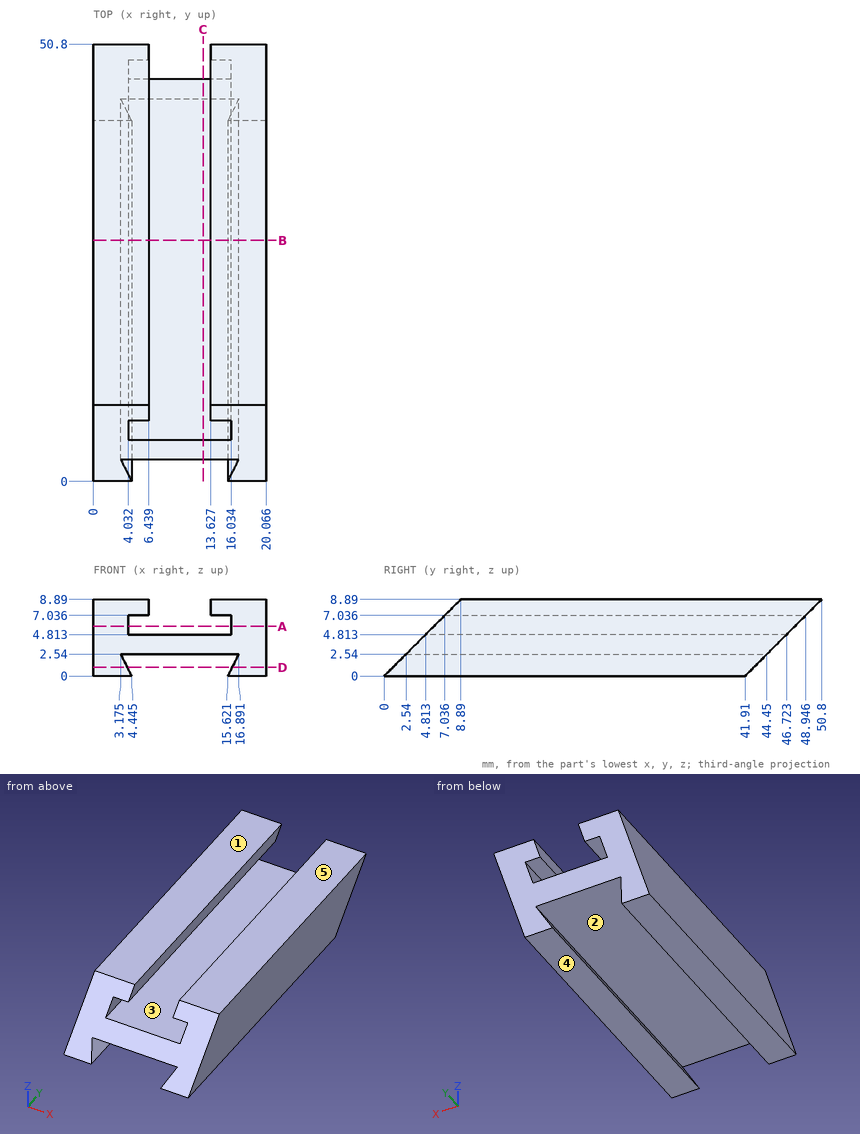
Source: three-view drawing plus pictorial views. Frame: mm from the lowest corner of the part. A direction names the side the tool comes from. Round coordinates to 2 decimals unless told otherwise and drop trailing zeros. Write each loop counter-clockwise with the first axis right and the second up, starting at its lowest first coordinate (ties: lowest second). Pieces come first, ordered by that corner, then holes. Notation, with made-up numbers: M -12.5,40.5 L -8.5,40.5 A26 ccw -8.5,70.5 Z; hole C 30.5,73.5 d3. An arc over 180 degrees is marked long. One line per item, written item: value. Start each with the question number.
Item 1: Section query D-D (z = 1). Return the cut outline in (x, y) (1 decimal), plus the area to 3 significant figures.
Item 2: Section query C-C (x = 12.75). Return the cut outline in (y, z).
Item 3: Section query B-B (y = 28). Return the cut outline in (x, z) (1 decimal).
Item 4: Section query A-A (z = 5.75). Return the cut outline in (x, y), plus the area to 3 significant figures.
Item 5: Pin query (flat end, axial travel): pin 1 (4 mm diameter, centred on x = 9.5, y = 19.5, fed in from +Z); pin 2 (1.5 mm diameter, centred on x = 15.5, z = 7.5, fed in from +Y). Return the tip coordinate at first contact, or that it passes through.
Item 6: Ray query, L1, parallel to Z at x = 15.5, y = 18.5; L2, parallel to X at y = 18, z = 5.25; L3, parallel to Z at x = 4.25, y = 8.5 (1 decimal). Return the intervals inside material, ascending. Write a range as from..to.
Item 7: Mould query, pull axis Z, two halves, no side actions, for the marked faces 3, 4 and 5. Classes: pulls with the +Z half, pulls with the -Z half, needs draft (parallel to the pull), parting line crosses it, or undercut.
Item 8: Set-up query: the marked faces 1 and 2. Return all of +Z, -Z, +X, -X, +Y, -Y with unobstructed straight access to the full face (end or side cutting, diameter ignored); none if empty.
Result set:
1. outline: M 0,1 L 3.9,1 L 3.9,42.9 L 0,42.9 Z; M 16.1,1 L 20.1,1 L 20.1,42.9 L 16.1,42.9 Z
1. area: 331 mm²
2. outline: M 2.54,2.54 L 44.45,2.54 L 46.72,4.81 L 4.81,4.81 Z
3. outline: M 0,0 L 4.4,0 L 3.2,2.5 L 16.9,2.5 L 15.6,0 L 20.1,0 L 20.1,8.9 L 13.6,8.9 L 13.6,7 L 16,7 L 16,4.8 L 4,4.8 L 4,7 L 6.4,7 L 6.4,8.9 L 0,8.9 Z
4. outline: M 0,5.75 L 4.03,5.75 L 4.03,47.66 L 0,47.66 Z; M 16.03,5.75 L 20.07,5.75 L 20.07,47.66 L 16.03,47.66 Z
4. area: 338 mm²
5. pin 1: stops at z = 4.81
5. pin 2: stops at y = 50.16
6. L1: z = 2.54..4.81, 7.04..8.89
6. L2: x = 0..4.03, 16.03..20.07
6. L3: z = 0..0.4, 2.5..4.8, 7..8.5
7. face 3: undercut
7. face 4: pulls with the -Z half
7. face 5: pulls with the +Z half
8. face 1: +Z, +X, -X, +Y, -Y
8. face 2: +Y, -Y
